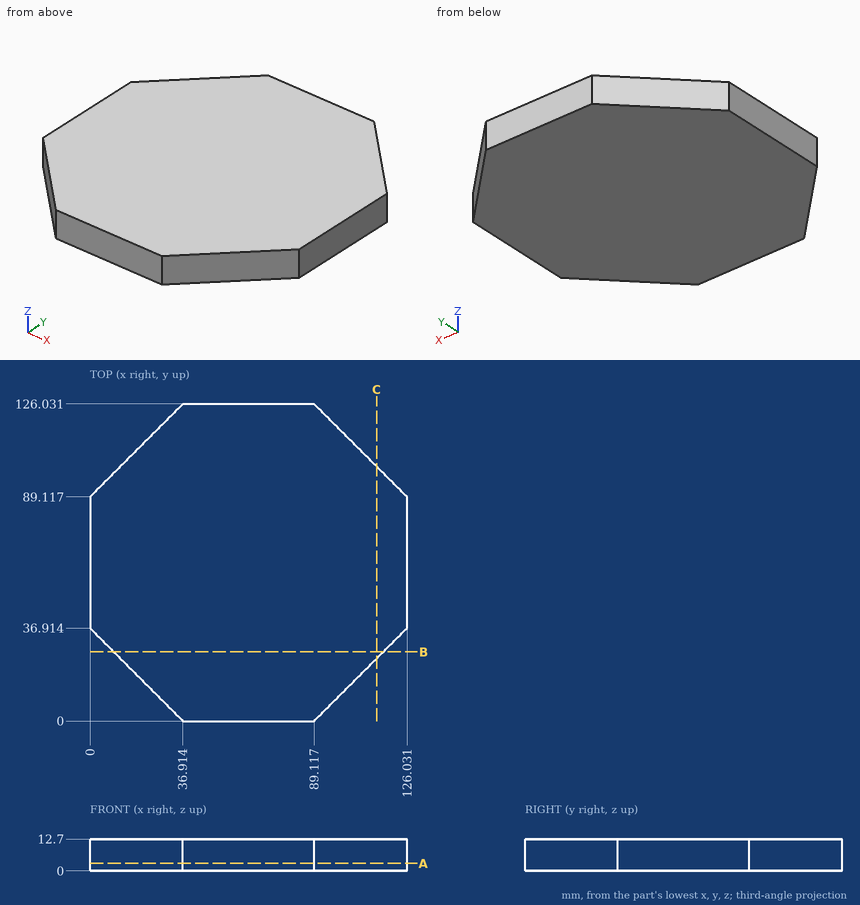
The drawing under review shows one solid part. Ordinate dimensions are in mm from its lowest x, y, z. Give positions to 0.01 mm unless a question says otherwise; leave off trailing zeros. Write each loop counter-clockwise with the first axis right and the second up, starting at its lowest first coordinate (ties: lowest second). Pieces come first, ordered by that corner, then holes. Notation, with made-up numbers: (2, 56) -> (6, 56) arc R23 cw to (6, 93) -> close; hole circle Ø9 at (49, 45). An arc over 180 degrees is marked (long way). Put each result on its own line as item: value.
(1) To check wall thickness, follow probe 1 along X at (y, z) = (17.5, 12) (1 decimal); probe 2 along X at (y, z) = (35, 11) (1 decimal); probe 3 along Y at (x, z) = (8, 4.5) (1 decimal). State the ranges of each line that lie inside material, in increasing order. Write a range as from..to.
Results are:
probe 1: 19.4..106.6
probe 2: 1.9..124.1
probe 3: 28.9..97.1
(2) We need section A-A, the plane z = 3. Give the boundary of the cut face in (x, y), and give its area (3 significant figures).
Results are:
outline: (0, 36.91) -> (36.91, 0) -> (89.12, 0) -> (126.03, 36.91) -> (126.03, 89.12) -> (89.12, 126.03) -> (36.91, 126.03) -> (0, 89.12) -> close
area: 13,200 mm²
(3) We need section C-C, the plane x = 114. Give the boundary of the cut face in (y, z).
Results are:
outline: (24.88, 0) -> (101.15, 0) -> (101.15, 12.7) -> (24.88, 12.7) -> close
(4) For pin 1 Ø5 at (y, z) = (67.5, 2) entering from -X, flat-tipped, find the tip position at first contact; note if it passes through.
Results are:
pin 1: x = 0
(5) We need section B-B, the plane y = 27.5. Give the boundary of the cut face in (x, z).
Results are:
outline: (9.41, 0) -> (116.62, 0) -> (116.62, 12.7) -> (9.41, 12.7) -> close
